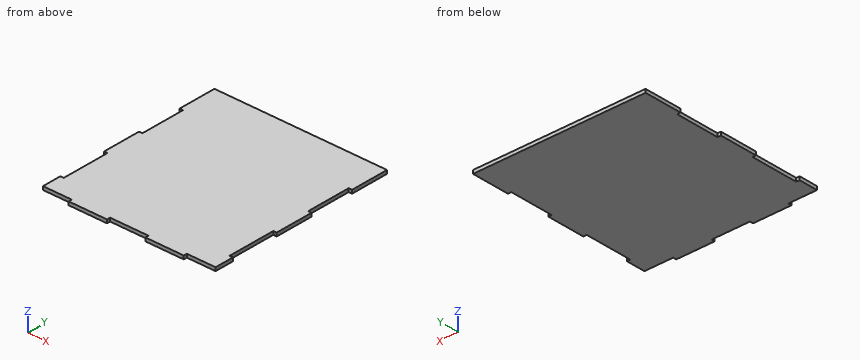
Solid Edge part; units mm, degrees
sketch "Sketch1" plane through (0, 0, 0) normal (0, 0, 1) x (1, 0, 0)
  line L0 (-114.3, -127) -> (114.3, -127)
  line L1 (114.3, -127) -> (114.3, 127)
  line L2 (114.3, 127) -> (-114.3, 127)
  line L3 (-114.3, 127) -> (-114.3, -127)
  dimension "D1" = 114.3
  dimension "D2" = 114.3
extrude "Protrusion1" add sketch "Sketch1" along normal blind 4.4958
sketch "Sketch2" plane through (0, 0, 4.4958) normal (0, 0, 1) x (1, 0, 0)
  line L0 (-76.2, -122.5042) -> (-76.2, -127)
  line L1 (-114.3, -127) -> (-76.2, -127)
  line L2 (-114.3, -122.5042) -> (-114.3, -127)
  line L3 (-76.2, -122.5042) -> (-114.3, -122.5042)
  line L4 (25.4, -122.5042) -> (-25.4, -122.5042)
  line L5 (-25.4, -122.5042) -> (-25.4, -127)
  line L6 (-25.4, -127) -> (25.4, -127)
  line L7 (25.4, -122.5042) -> (25.4, -127)
  line L8 (76.2, -122.5042) -> (76.2, -127)
  line L9 (76.2, -127) -> (114.3, -127)
  line L10 (114.3, -127) -> (114.3, -122.5042)
  line L11 (114.3, -122.5042) -> (76.2, -122.5042)
extrude "Cutout1" cut sketch "Sketch2" against normal through all
sketch "Sketch3" plane through (0, 0, 4.4958) normal (0, 0, 1) x (1, 0, 0)
  line L0 (-109.8042, -97.1042) -> (-109.8042, -33.6042)
  line L1 (-109.8042, -33.6042) -> (-114.3, -33.6042)
  line L2 (-114.3, -33.6042) -> (-114.3, -97.1042)
  line L3 (-109.8042, -97.1042) -> (-114.3, -97.1042)
  line L4 (-114.3, 76.2) -> (-114.3, 17.1958)
  line L5 (-109.8042, 17.1958) -> (-114.3, 17.1958)
  line L6 (-109.8042, 17.1958) -> (-109.8042, 76.2)
  line L7 (-109.8042, 76.2) -> (-114.3, 76.2)
extrude "Cutout2" cut sketch "Sketch3" against normal through all
mirror "Mirror1" about plane through (0, 0, 0) normal (-1, 0, 0) of "Cutout2"
properties material "Acrylic, high impact grade"
CAD build for the part. Positions are in the model's coordinates, mm. Round coordinates to 2 decimals unless told otherwise and drop trailing zeros. Order: outer loops, then holes, each group sorted by start corner. A loop starts at its lowest first (then second) coordinate and runs counter-clockwise, first axis right, second up. Notation, with made-up numbers: (2, 42.5) -> (14, 42.5) arc R7 cw to (14, 47.5) -> close; hole circle Ø2 at (60, 86.25). An arc over 180 degrees is marked (long way). Write item = value, one per line.
(1) Cut at A-A (z = 3). Write the cut outline in (x, y).
Answers follow:
outline = (-114.3, -122.5) -> (-76.2, -122.5) -> (-76.2, -127) -> (-25.4, -127) -> (-25.4, -122.5) -> (25.4, -122.5) -> (25.4, -127) -> (76.2, -127) -> (76.2, -122.5) -> (114.3, -122.5) -> (114.3, -97.1) -> (109.8, -97.1) -> (109.8, -33.6) -> (114.3, -33.6) -> (114.3, 17.2) -> (109.8, 17.2) -> (109.8, 76.2) -> (114.3, 76.2) -> (114.3, 127) -> (-114.3, 127) -> (-114.3, 76.2) -> (-109.8, 76.2) -> (-109.8, 17.2) -> (-114.3, 17.2) -> (-114.3, -33.6) -> (-109.8, -33.6) -> (-109.8, -97.1) -> (-114.3, -97.1) -> close
(2) Flat gauge pins, fed straight in: P1, Ø2, axis at y = -125, z = 1.5, coming from the -X side; P2, Ø2, axis at y = 73.5, z = 2, coming from the +X side; P3, Ø2, axis at x = -113, z = 1.5, coming from the -Y side. Where does each tip first touch, or does it go through?
Answers follow:
P1 = -76.2
P2 = 109.8
P3 = -122.5
(3) Cut at B-B (y = -80). Write the cut outline in (x, z), plus the area to 3 significant figures.
Answers follow:
outline = (-109.8, 0) -> (109.8, 0) -> (109.8, 4.5) -> (-109.8, 4.5) -> close
area = 987 mm²
(4) Drill centre lines: L1, parallel to Y at x = 9, z = 0.9; L2, parallel to X at y = 46, z = 1.7. Where is each one in solid material? Low to high.
Answers follow:
L1 = -122.5 to 127
L2 = -109.8 to 109.8
